```python
from build123d import *

# Parameters (mm, degrees)
SKETCH_1_W      = 10.5
SKETCH_1_H      = 3.5
SKETCH_1_W_2    = 3.5
SKETCH_1_H_2    = 5.5
SKETCH_1_W_3    = 3.520169939
EXTRUDE_1_DEPTH = 3


with BuildPart() as part:
    # Эскиз1 → Бобышка-Вытянуть1 (new body)
    with BuildSketch(Plane.XY):
        Polygon((-27.25, 30), (27.25, 30), (27.25, 19.75), (30.75, 19.75), (30.75, 30), (33, 30), (33, -30), (30.816819074, -30), (30.816819074, -19.75), (27.296649135, -19.75), (27.296649135, -30), (-27.296649135, -30), (-27.296649135, -19.75), (-30.816819074, -19.75), (-30.816819074, -30), (-33, -30), (-33, 30), (-30.75, 30), (-30.75, 19.75), (-27.25, 19.75), align=None)
        with Locations((-12.5, 16)):
            Rectangle(SKETCH_1_W, SKETCH_1_H, mode=Mode.SUBTRACT)
        with Locations((-29, 7.5)):
            Rectangle(SKETCH_1_W_2, SKETCH_1_H_2, mode=Mode.SUBTRACT)
        with Locations((-29.056734105, -7.5)):
            Rectangle(SKETCH_1_W_3, SKETCH_1_H_2, mode=Mode.SUBTRACT)
        with Locations((29.056734105, -7.5)):
            Rectangle(SKETCH_1_W_3, SKETCH_1_H_2, mode=Mode.SUBTRACT)
        with Locations((29, 7.5)):
            Rectangle(SKETCH_1_W_2, SKETCH_1_H_2, mode=Mode.SUBTRACT)
        with Locations((12.5, 16)):
            Rectangle(SKETCH_1_W, SKETCH_1_H, mode=Mode.SUBTRACT)
    extrude(amount=EXTRUDE_1_DEPTH)


solid = part.part
```
Geometry: final body of the model. Coordinates: model frame, mm. A direction names the side the tool comes from. Round coordinates to 2 decimals unless told otherwise and drop trailing zeros. Loops run counter-clockwise (first coordinate to the right, second up) from the corner with the lowest first, then second, coordinate; pieces in that order, holes last. Notation, with made-up numbers: (-22, 30.25) -> (35, 30.25) arc R25 cw to (35, 68.25) -> close; hole circle Ø9 at (24.5, 11). An arc over 180 degrees is marked (long way). Use one line per item in the form item = value.
Item 1: Cut plane C-C on y = -8. Output: boundary loops of the cut face in (x, z).
Evaluation:
outline = (-33, 0) -> (-30.82, 0) -> (-30.82, 3) -> (-33, 3) -> close; (-27.3, 0) -> (27.3, 0) -> (27.3, 3) -> (-27.3, 3) -> close; (30.82, 0) -> (33, 0) -> (33, 3) -> (30.82, 3) -> close
Item 2: Draft query along X for faces 1 (the flat face through (-27.25, 7, 1)), 2 (the flat face through (0, -30, 1)). Return one class per face: released by +X, released by -X, zero draft, split by the parting line, or undercut.
Evaluation:
face_1 = undercut
face_2 = zero draft
Item 3: Cut plane A-A on y = 21. Output: boundary loops of the cut face in (x, z).
Evaluation:
outline = (-33, 0) -> (-30.75, 0) -> (-30.75, 3) -> (-33, 3) -> close; (-27.25, 0) -> (27.25, 0) -> (27.25, 3) -> (-27.25, 3) -> close; (30.75, 0) -> (33, 0) -> (33, 3) -> (30.75, 3) -> close
Item 4: Cut plane D-D on z = 0.8. Give the number of separate pieces and of enclosed holes in the cut face, then the cut area to 3 significant figures.
Evaluation:
separate_pieces = 1
enclosed_holes = 6
area = 3,670 mm2
Item 5: Contact query for flat-ended pins moving along their axis: pin 1 Ø1.5 at (x, z) = (29, 1) entering from +Y; pin 2 Ø0.9 at (x, z) = (29, 1.5) entering from -Y. Output: stop coordinate, or through.
Evaluation:
pin_1 = 19.75
pin_2 = -19.75
Item 6: Cut plane B-B on x = -15.5. Output: boundary loops of the cut face in (y, z).
Evaluation:
outline = (-30, 0) -> (14.25, 0) -> (14.25, 3) -> (-30, 3) -> close; (17.75, 0) -> (30, 0) -> (30, 3) -> (17.75, 3) -> close
Item 7: Material intervals for probe 1 along X at (y, z) = (-20, 1.3); probe 2 along X at (y, z) = (25, 1.3); probe 3 along Y at (x, z) = (30, 2.25), sorted ascending.
Evaluation:
probe_1 = -33 to -30.82, -27.3 to 27.3, 30.82 to 33
probe_2 = -33 to -30.75, -27.25 to 27.25, 30.75 to 33
probe_3 = -19.75 to -10.25, -4.75 to 4.75, 10.25 to 19.75
Item 8: Access query for faces 3 (the flat face through (29, 10.25, 1)), 4 (the flat face through (27.297, -25, 1)), 5 (the flat face through (-27.25, 25, 1)). Directions: +Z, -Z, +X, -X, +Y, -Y. A direction counts if a zero-diameter tool reaches every point of the face in a straight line with its end or side. Return the directions, or none.
Evaluation:
face_3 = +Z, -Z
face_4 = +Z, -Z, -Y
face_5 = +Z, -Z, +Y
